Read the model definition and answer for the solid it produces. Units are mm, in the model's axes. Face numbers are marked on the shaded views. A direction names the side the tool comes from. Give positions to 0.01 mm unless a question says otherwise; leave off trailing zeros. Write each loop counter-clockwise with the first axis right and the second up, starting at its lowest first coordinate (ties: lowest second). Pieces come first, ordered by that corner, then holes. Notation, with made-up numbers: (87.25, 65) -> (144.25, 65) arc R19 cw to (144.25, 85) -> close; hole circle Ø10 at (1, 5.5). An arc over 180 degrees is marked (long way). Use a Markdown table: item, result.
Autodesk Inventor part; units mm, degrees
ref_plane "YZ Plane" through (0, 0, 0) normal (1, 0, 0) x (0, 1, 0)
ref_plane "XZ Plane" through (0, 0, 0) normal (0, 1, 0) x (-1, 0, 0)
ref_plane "XY Plane" through (0, 0, 0) normal (0, 0, 1) x (1, 0, 0)
sketch "스케치3" plane through (0, 0, 0) normal (0, 1, 0) x (-1, 0, 0)
  line L0 (19.4959, -8.0755) -> (8.0755, -19.4959)
  line L1 (8.0755, -19.4959) -> (-8.0755, -19.4959)
  line L2 (-8.0755, -19.4959) -> (-19.4959, -8.0755)
  line L3 (-19.4959, -8.0755) -> (-19.4959, 8.0755)
  line L4 (-19.4959, 8.0755) -> (-8.0755, 19.4959)
  line L5 (-8.0755, 19.4959) -> (8.0755, 19.4959)
  line L6 (8.0755, 19.4959) -> (19.4959, 8.0755)
  line L7 (19.4959, 8.0755) -> (19.4959, -8.0755)
  line L8 (6.75, -16.2959) -> (-6.75, -16.2959)
  line L9 (-6.75, -16.2959) -> (-16.2959, -6.75)
  line L10 (-16.2959, -6.75) -> (-16.2959, 6.75)
  line L11 (-16.2959, 6.75) -> (-6.75, 16.2959)
  line L12 (-6.75, 16.2959) -> (6.75, 16.2959)
  line L13 (6.75, 16.2959) -> (16.2959, 6.75)
  line L14 (16.2959, 6.75) -> (16.2959, -6.75)
  line L15 (16.2959, -6.75) -> (6.75, -16.2959)
  point P0 (0, 0)
  point P1 (0, 0)
  point P2 (0, 0)
  point P3 (0, 0)
  dimension "d66" = 13.5
  dimension "d67" = 3.2
extrude "돌출2" add sketch "스케치3" along normal blind 3.4 contours L0 L1 L2 L3 L4 L5 L6 L7 | L8 L9 L10 L11 L12 L13 L14 L15
sketch "스케치9" plane through (0, 0, 0) normal (0, -1, 0) x (1, 0, 0)
  line L0 (7.5, 10) -> (2.5, 10)
  line L1 (2.5, 10) -> (2.5, -10)
  line L2 (2.5, -10) -> (7.5, -10)
  line L3 (7.5, -10) -> (7.5, 10)
  line L4 (7.5, 10) -> (2.5, -10) construction
  line L5 (2.5, 10) -> (7.5, -10) construction
  line L6 (-2.5, 10) -> (-7.5, 10)
  line L7 (-7.5, 10) -> (-7.5, -10)
  line L8 (-7.5, -10) -> (-2.5, -10)
  line L9 (-2.5, 10) -> (-7.5, -10) construction
  line L10 (-7.5, 10) -> (-2.5, -10) construction
  line L11 (-2.5, -10) -> (-2.5, 10)
  point P0 (0, 0)
  point P1 (5, 0)
  point P2 (-5, 0)
  dimension "d42" = 20
  dimension "d43" = 5
  dimension "d44" = 2.5
  dimension "d47" = 10
extrude "돌출8" add sketch "스케치9" along normal blind 10
sketch "스케치10" plane through (-7.5, 0, -10) normal (-1, 0, 0) x (0, 0, 1)
  circle A0 centre (15, -5) radius 1.25
  line L0 (19.9591, 0) -> (0.0886, 0)
  line L1 (18.0755, 0) -> (1.9245, 0)
  circle A1 centre (5, -5) radius 1.25
  line L2 (20, 0) -> (20, -10)
  point P0 (10, 0)
  dimension "d54" = 2.5
  dimension "d57" = 10
  dimension "d62" = 5
  dimension "d63" = 5
extrude "돌출9" cut sketch "스케치10" against normal blind 20
fillet "모깎기1" radius 1.2 16 edges at (-13.7857, 3.4, 13.7857) (0, 3.4, 19.4959) (13.7857, 3.4, 13.7857) (19.4959, 3.4, 0) (13.7857, 3.4, -13.7857) (0, 3.4, -19.4959) (-13.7857, 3.4, -13.7857) (-19.4959, 3.4, 0) (-13.7857, 0, 13.7857) (0, 0, 19.4959) (13.7857, 0, 13.7857) (19.4959, 0, 0) (13.7857, 0, -13.7857) (0, 0, -19.4959) (-13.7857, 0, -13.7857) (-19.4959, 0, 0)
sketch "스케치12" plane through (0, 3.4, 0) normal (0, 1, 0) x (1, 0, 0)
  line L0 (7.4127, -17.8959) -> (-7.4127, -17.8959)
  line L1 (-7.4127, -17.8959) -> (-17.8959, -7.4127)
  line L2 (-17.8959, -7.4127) -> (-17.8959, 7.4127)
  line L3 (-17.8959, 7.4127) -> (-7.4127, 17.8959)
  line L4 (-7.4127, 17.8959) -> (7.4127, 17.8959)
  line L5 (7.4127, 17.8959) -> (17.8959, 7.4127)
  line L6 (17.8959, 7.4127) -> (17.8959, -7.4127)
  line L7 (17.8959, -7.4127) -> (7.4127, -17.8959)
  line L8 (-6.5843, 15.8959) -> (6.5843, 15.8959)
  line L9 (6.5843, 15.8959) -> (15.8959, 6.5843)
  line L10 (15.8959, 6.5843) -> (15.8959, -6.5843)
  line L11 (15.8959, -6.5843) -> (6.5843, -15.8959)
  line L12 (6.5843, -15.8959) -> (-6.5843, -15.8959)
  line L13 (-6.5843, -15.8959) -> (-15.8959, -6.5843)
  line L14 (-15.8959, -6.5843) -> (-15.8959, 6.5843)
  line L15 (-15.8959, 6.5843) -> (-6.5843, 15.8959)
  line L16 (-18.2959, -7.5784) -> (-18.2959, 7.5784)
  line L17 (-19.4959, 8.0755) -> (-19.4959, -8.0755)
  point P0 (0, 0)
  point P1 (0, 0)
  point P2 (0, 0)
  point P3 (-17.8959, 0)
  point P4 (-19.4959, 0)
  point P5 (-15.8959, 0)
  dimension "d100" = 1.6
  dimension "d101" = 2
extrude "돌출11" cut sketch "스케치12" against normal blind 1.2
sketch "스케치13" plane through (0, 3.4, 0) normal (0, 1, 0) x (1, 0, 0)
  line L0 (15.8959, 6.5843) -> (6.5843, 15.8959)
  line L1 (6.5843, 15.8959) -> (-6.5843, 15.8959)
  line L2 (-6.5843, 15.8959) -> (-15.8959, 6.5843)
  line L3 (-15.8959, 6.5843) -> (-15.8959, -6.5843)
  line L4 (-15.8959, -6.5843) -> (-6.5843, -15.8959)
  line L5 (-6.5843, -15.8959) -> (6.5843, -15.8959)
  line L6 (6.5843, -15.8959) -> (15.8959, -6.5843)
  line L7 (15.8959, -6.5843) -> (15.8959, 6.5843)
  point P0 (0, 0)
extrude "돌출12" cut sketch "스케치13" against normal blind 0.6
properties part number "OV-PAM_bottom_2"
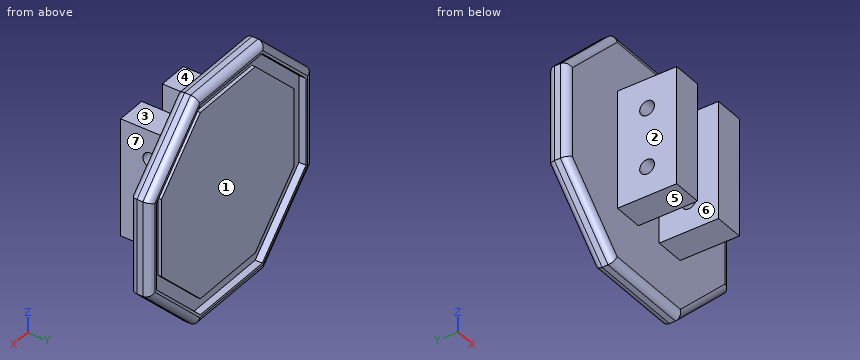
Item 1: A tool of negligible diameter and unlimited length cuts with its end or side. For the marked faces 4, 5, 6 and 7, from which of +Z, -Z, +X, -X, +Y, -Y can it reach the whole face along a straight path? Write none if from no direction.
Return value:
| item | result |
|---|---|
| face 4 | +Z, +X, -X, -Y |
| face 5 | -Z, +X, -X, -Y |
| face 6 | +Z, -Z, -Y |
| face 7 | +Z, -Z, +X, -Y |
Item 2: A cutting plane is placed at C-C (x = 6). Give the vertices of the cut face in (y, z).
Return value:
| item | result |
|---|---|
| outline | (-10, -10) -> (0, -10) -> (0, -18.3) arc R1.2 ccw to (1.2, -19.5) -> (2.2, -19.5) arc R1.2 ccw to (3.4, -18.3) -> (3.4, -17.9) -> (2.2, -17.9) -> (2.2, -15.9) -> (2.8, -15.9) -> (2.8, 15.9) -> (2.2, 15.9) -> (2.2, 17.9) -> (3.4, 17.9) -> (3.4, 18.3) arc R1.2 ccw to (2.2, 19.5) -> (1.2, 19.5) arc R1.2 ccw to (0, 18.3) -> (0, 10) -> (-10, 10) -> close; hole circle Ø2.5 at (-5, -5); hole circle Ø2.5 at (-5, 5) |
Item 3: Straight lines are drawn through the part: line 1 along Y through (x, z) = (-4, 5); line 2 along X through (y, z) = (-6.5, -5); line 3 along Z through (x, y) = (-5, -4.25). For each, find the intervals that lie inside material, in ascending order. Write a range as [from, to].
Return value:
| item | result |
|---|---|
| line 1 | [-10, -6.25], [-3.75, 2.8] |
| line 2 | [-7.5, -2.5], [2.5, 7.5] |
| line 3 | [-10, -6], [-4, 4], [6, 10] |
Item 4: A cutting plane is placed at D-D (y = -5). Give the vertices of the cut face in (x, z), then the cut area to 3 significant figures.
Return value:
| item | result |
|---|---|
| outline | (-7.5, -10) -> (-2.5, -10) -> (-2.5, -6.25) -> (-7.5, -6.25) -> close; (-7.5, -3.75) -> (-2.5, -3.75) -> (-2.5, 3.75) -> (-7.5, 3.75) -> close; (-7.5, 6.25) -> (-2.5, 6.25) -> (-2.5, 10) -> (-7.5, 10) -> close; (2.5, -10) -> (7.5, -10) -> (7.5, -6.25) -> (2.5, -6.25) -> close; (2.5, -3.75) -> (7.5, -3.75) -> (7.5, 3.75) -> (2.5, 3.75) -> close; (2.5, 6.25) -> (7.5, 6.25) -> (7.5, 10) -> (2.5, 10) -> close |
| area | 150 mm^2 |
Item 5: A cutting plane is placed at A-A (z = -5). Count the separate pieces of the cut face and the enclosed holes in it, then the cut area to 3 significant figures.
Return value:
| item | result |
|---|---|
| separate pieces | 3 |
| enclosed holes | 0 |
| area | 182 mm^2 |
Item 6: For a pull along X with two mould halves and no side action, classify the marked faces 1, 2 and 3 as +X half, -X half, draft (parallel to the pull), parting line (faces both ways), or undercut.
Return value:
| item | result |
|---|---|
| face 1 | undercut |
| face 2 | -X half |
| face 3 | draft |
Item 7: Each of these flat-tipped pins is pushed along its axis until it touches: P1, Ø8, axis at y = -4.5, z = 1, coming from the +X side; P2, Ø6, axis at x = -8, y = 1, coming from the -Z side; P3, Ø3, axis at y = -3.5, z = -8.5, coming from the -X side; P4, Ø1.5, axis at y = -5, z = 5, coming from the -X side. Where does it stop, or does it pass through?
Return value:
| item | result |
|---|---|
| P1 | x = 7.5 |
| P2 | z = -19.5 |
| P3 | x = -7.5 |
| P4 | through |
Item 8: A cutting plane is placed at B-B (y = -0.75). Give the vertices of the cut face in (x, z), then the cut area to 3 significant figures.
Return value:
| item | result |
|---|---|
| outline | (-7.5, -10) -> (-2.5, -10) -> (-2.5, 10) -> (-7.5, 10) -> close; (2.5, -10) -> (7.5, -10) -> (7.5, 10) -> (2.5, 10) -> close |
| area | 200 mm^2 |
